from build123d import *

# Parameters (mm, degrees)
SKETCH3_W                = 1016
SKETCH3_H                = 609.6
SKETCH3_W_2              = 965.2
SKETCH3_H_2              = 558.8
BOSS_EXTRUDE1_DEPTH      = 25.4
SKETCH4_W                = 25.4
SKETCH4_H                = 25.4
BOSS_EXTRUDE2_DEPTH      = 228.6
BOSS_EXTRUDE3_DEPTH      = 330.2
BOSS_EXTRUDE3_DEPTH_BACK = 25.4
SKETCH6_W                = 25.4
SKETCH6_H                = 25.4
BOSS_EXTRUDE4_DEPTH      = 431.8
BOSS_EXTRUDE4_DEPTH_BACK = 25.4
SKETCH7_W                = 25.4
SKETCH7_H                = 25.4
SKETCH8_W                = 25.4
SKETCH8_H                = 25.4
BOSS_EXTRUDE5_DEPTH      = 558.8


with BuildPart() as part:
    # Sketch3 → Boss-Extrude1 (new body)
    with BuildSketch(Plane(origin=(0, 0, 0), x_dir=(1, 0, 0), z_dir=(0, 1, 0))):
        Rectangle(SKETCH3_W, SKETCH3_H)
        Rectangle(SKETCH3_W_2, SKETCH3_H_2, mode=Mode.SUBTRACT)
    extrude(amount=BOSS_EXTRUDE1_DEPTH)

    # Sketch4 → Boss-Extrude2 (add)
    with BuildSketch(Plane(origin=(0, 25.4, 0), x_dir=(1, 0, 0), z_dir=(0, 1, 0))):
        with Locations((-495.3, 292.1)):
            Rectangle(SKETCH4_W, SKETCH4_H)
        with Locations((495.3, 292.1)):
            Rectangle(SKETCH4_W, SKETCH4_H)
        with Locations((495.3, -292.1)):
            Rectangle(SKETCH4_W, SKETCH4_H)
        with Locations((-495.3, -292.1)):
            Rectangle(SKETCH4_W, SKETCH4_H)
    extrude(amount=BOSS_EXTRUDE2_DEPTH)

    # Sketch6 → Boss-Extrude3 (add, two sides: drawn at the far end of the back side and taken through both)
    with BuildSketch(Plane(origin=(-482.6, 0, 0), x_dir=(0, 0, -1), z_dir=(1, 0, 0)).offset(-BOSS_EXTRUDE3_DEPTH_BACK)):
        with Locations((-292.1, 266.7)):
            Rectangle(SKETCH6_W, SKETCH6_H)
        with Locations((292.1, 266.7)):
            Rectangle(SKETCH6_W, SKETCH6_H)
    extrude(amount=BOSS_EXTRUDE3_DEPTH + BOSS_EXTRUDE3_DEPTH_BACK)

    # Sketch7 → Boss-Extrude4 (add, two sides: drawn at the far end of the back side and taken through both)
    with BuildSketch(Plane.ZY.offset(-482.6).offset(-BOSS_EXTRUDE4_DEPTH_BACK)):
        with Locations((292.1, 266.7)):
            Rectangle(SKETCH7_W, SKETCH7_H)
        with Locations((-292.1, 266.7)):
            Rectangle(SKETCH7_W, SKETCH7_H)
    extrude(amount=BOSS_EXTRUDE4_DEPTH + BOSS_EXTRUDE4_DEPTH_BACK)

    # Sketch8 → Boss-Extrude5 (add)
    with BuildSketch(Plane.XY.offset(-279.4)):
        with Locations((495.3, 266.7)):
            Rectangle(SKETCH8_W, SKETCH8_H)
        with Locations((-495.3, 266.7)):
            Rectangle(SKETCH8_W, SKETCH8_H)
    extrude(amount=BOSS_EXTRUDE5_DEPTH)


solid = part.part
Here's how the part is built. I have some questions about the finished solid (model axes, mm). A direction names the side the tool comes from. Coordinates: 2 decimals unless noted, no trailing zeros. Order: outer loops, then holes, each group sorted by start corner. A loop starts at its lowest first (then second) coordinate and runs counter-clockwise, first axis right, second up. Notation, with made-up numbers: M -39.5,-13 L -20.5,-13 A13 ccw -20.5,12 Z; hole C 77.25,-8 d11. An arc over 180 degrees is marked long. Answer as CSV lines item,"result". Start each with the question number.
1. For pin 1 (7.5 mm diameter, centred on x = -140.5, z = 297.5, fed in from +Y), with a flat end and sliding along its axis, tell me the tip position at first contact or that it passes through.
2. I want a section at A-A, the plane z = -197.5. Write out the boundary of the cut face in (x, y).
3. On a 3-axis mill with a long thin cutter (end or side, diameter ignored), from which of +Z, -Z, +X, -X, +Y, -Y can I reach the whole of each face in a straight line? I mean faces 5 (the flat face through (-7, 25.4, -292)), 6 (the flat face through (-508, 254.2, -21.2)), 7 (the flat face through (50.8, 267, -292)), 8 (the flat face through (482.6, 13, 4)). Say none if no direction works.
4. We'd pull the mould along Z, two halves only. Please class faces 1 (the flat face through (-2, 25, -304.8)), 2 (the flat face through (-495, 25.4, -4)), 3 (the flat face through (482.6, 267, -4)), 4 (the flat face through (-152.4, 267, 292)): released by +Z, released by -Z, zero draft, split by the parting line, or undercut.
5. I want a section at B-B, the plane x = -400. Write out the boundary of the cut face in (y, z), and give its area (3 significant figures).
6. I need wall thicknesses on line 1 (Z direction, x = -369.5, y = 20); line 2 (X direction, y = 256.5, z = -27). Which ranges of each line are inside material? Lowest first, please. Write a range as [from, to].
Recorded:
1,pin 1,"stops at y = 25.4"
2,outline,"M -508,0 L -482.6,0 L -482.6,25.4 L -508,25.4 Z; M -508,254 L -482.6,254 L -482.6,279.4 L -508,279.4 Z; M 482.6,0 L 508,0 L 508,25.4 L 482.6,25.4 Z; M 482.6,254 L 508,254 L 508,279.4 L 482.6,279.4 Z"
3,face 5,"+Z, -Z"
3,face 6,"+Z, -Z, -X, +Y, -Y"
3,face 7,"+Z, -Z, +Y"
3,face 8,"+Y, -Y"
4,face 1,"released by -Z"
4,face 2,"undercut"
4,face 3,"undercut"
4,face 4,"zero draft"
5,outline,"M 0,-304.8 L 25.4,-304.8 L 25.4,-279.4 L 0,-279.4 Z; M 0,279.4 L 25.4,279.4 L 25.4,304.8 L 0,304.8 Z; M 254,-304.8 L 279.4,-304.8 L 279.4,-279.4 L 254,-279.4 Z; M 254,279.4 L 279.4,279.4 L 279.4,304.8 L 254,304.8 Z"
5,area,"2,580 mm2"
6,line 1,"z = [-304.8, -279.4], [279.4, 304.8]"
6,line 2,"x = [-508, -482.6], [482.6, 508]"
